```python
from build123d import *

# Parameters (mm, degrees)
F1_DEPTH = 20.3326418996
F1_TAPER = 7
F2_SIZE  = 1


with BuildPart() as f1:
    # F0 (on Top) → F1 (new body)
    with BuildSketch(Plane.XY):
        Polygon((3.2104404383, -5.701944282), (6.5432488184, -0.0706491641), (3.3328083801, 5.6312951179), (-3.2104404383, 5.701944282), (-6.5432488184, 0.0706491641), (-3.3328083801, -5.6312951179), align=None)
    extrude(amount=F1_DEPTH, taper=F1_TAPER)

    # F2
    f2_edges = [f1.edges().sort_by_distance(p)[0] for p in [
        (2.762615, 1.555471, 20.332642),
        (-2.762615, -1.555471, 20.332642),
        (0.03423, 3.170231, 20.332642),
        (-2.728385, 1.614759, 20.332642),
        (-0.03423, -3.170231, 20.332642),
        (2.728385, -1.614759, 20.332642),
    ]]
    chamfer(f2_edges, length=F2_SIZE)


solid = f1.part
```
For this review, take the finished solid that the model builds, in its own axes (mm). Round coordinates to 2 decimals unless told otherwise and drop trailing zeros. Order: outer loops, then holes, each group sorted by start corner. A loop starts at its lowest first (then second) coordinate and runs counter-clockwise, first axis right, second up.
Q1. We need section B-B, the plane z = 10.75. Give the boundary of the cut face in (x, y).
Findings below:
outline: (-5.02, 0.05) - (-2.56, -4.32) - (2.46, -4.37) - (5.02, -0.05) - (2.56, 4.32) - (-2.46, 4.37) - close
Q2. Wall thickness on line 1 (X direction, y = -3.25, z = 7); line 2 (X direction, y = -2, z = 3.75); line 3 (Y direction, x = -4.75, z = 5.75): over which ranges is each line inside the solid? List them lowest first.
Findings below:
line 1: x = -3.69 to 3.66
line 2: x = -4.85 to 4.87
line 3: y = -1.68 to 1.71
Q3. We need section A-A, the plane y = -2.75. Give the boundary of the cut face in (x, z), plus the area to 3 significant figures.
Findings below:
outline: (-4.96, 0) - (4.96, 0) - (2.2, 19.34) - (1.55, 19.83) - (-1.63, 19.8) - (-2.23, 19.34) - close
area: 140 mm2
Q4. We need section C-C, the plane x = -5. Give the boundary of the cut face in (y, z).
Findings below:
outline: (-2.67, 0) - (2.68, 0) - (0.05, 10.89) - close
Q5. Insertion check: P1, Ø1.5, axis at x = 4.5, y = -1.5, coming from the -Z side; P2, Ø1, axis at y = 4, z = 4, coming from the -X side; P3, Ø3, axis at x = 3, z = 14.5, coming from the +Y side; P4, Ø1, axis at x = -2, z = 2, coming from the +Y side. Each pin has a flat end and moves straight along its axis. Give the tip position at first contact, or say it passes through.
Findings below:
P1: stops at z = 0
P2: stops at x = -3.95
P3: stops at y = 4.03
P4: stops at y = 5.5
Q6. We need section D-D, the plane y = -5. Give the boundary of the cut face in (x, z).
Findings below:
outline: (-3.69, 0) - (3.63, 0) - (2.82, 5.68) - (-2.96, 5.17) - close
